Build history of the part. All positions in model axes, mm. Coordinates: 2 decimals unless noted, no trailing zeros. Write each loop counter-clockwise with the first axis right and the second up, starting at its lowest first coordinate (ties: lowest second). Pieces come first, ordered by that corner, then holes.
from build123d import *
from build123d.topology import SkipClean

# Parameters (mm, degrees)
SKETCH1_R           = 9.525
BOSS_EXTRUDE1_DEPTH = 25.4


with BuildPart() as part:
    # Sketch1 → Boss-Extrude1 (new body)
    with BuildSketch(Plane.XY):
        Circle(SKETCH1_R)
    extrude(amount=BOSS_EXTRUDE1_DEPTH)

    # Sketch2 → Revolve1 (revolve)
    with BuildSketch(Plane(origin=(0, 0, 0), x_dir=(0, 0, -1), z_dir=(1, 0, 0))):
        with BuildLine():
            Line((0, 9.525), (0, -9.525))
            ThreePointArc((0, -9.525), (9.525, 0), (0, 9.525))
        make_face()
    revolve(axis=Axis((0, 9.525, 0), (0, -1, 0)))

    # Sketch3 → Revolve2 (revolve)
    with SkipClean():  # the faces are left unmerged after this step: merging them gives an invalid solid
        with BuildSketch(Plane(origin=(0, 0, 0), x_dir=(0, 0, -1), z_dir=(1, 0, 0))):
            with BuildLine():
                Line((-25.4, 9.525), (-25.4, -9.525))
                ThreePointArc((-25.4, -9.525), (-34.925, 0), (-25.4, 9.525))
            make_face()
        revolve(axis=Axis((0, 9.525, 25.4), (0, -1, 0)))


solid = part.part
(1) Slice it at B-B, the plane z = 20. List the corners of the cut face in (x, y) (3 decimals), and give its area (3 significant figures).
(2) Slice it at D-D, the plane z = 28. List the corners of the cut face in (x, y), and give its area (3 significant figures).
(3) Slice it at A-A, the plane y = 0. List the corners of the cut face in (x, z) (3 decimals), and give its area (3 significant figures).
(4) Probe L1, parallel to Y at x = -2.5, z = 17.5; L2, parallel to Y at x = 3.5, z = -6; L3, parallel to X at y = -3.75, z = 33. List the from-to ranges inside material, lowest first.
(5) Flat gauge pins, fed straight in: P1, Ø6, axis at x = -0.5, z = 29, coming from the -Y side; P2, Ø1, axis at y = -7, z = 10, coming from the +X side; P3, Ø3, axis at y = -3.5, z = -2.5, coming from the -X side. Where does each tip first touch, or does it go through?
(6) Slice it at C-C, the plane x = 3. List the corners of the cut face in (y, z), and give its area (3 significant figures).
Results:
1. outline: circle Ø19.05 at (0, 0)
1. area: 285 mm2
2. outline: circle Ø18.33 at (0, 0)
2. area: 264 mm2
3. outline: (-9.525, 0) arc R9.525 ccw to (9.525, 0) - (9.525, 25.4) arc R9.525 ccw to (-9.525, 25.4) - close
3. area: 769 mm2
4. L1: y = -9.19 to 9.19
4. L2: y = -6.52 to 6.52
4. L3: x = -4.35 to 4.35
5. P1: stops at y = -9.5
5. P2: stops at x = 6.96
5. P3: stops at x = -9.1
6. outline: (-9.04, 0) arc R9.04 ccw to (9.04, 0) - (9.04, 25.4) arc R9.04 ccw to (-9.04, 25.4) - close
6. area: 716 mm2
